```python
from build123d import *

# Parameters (mm, degrees)
F0_W     = 60
F0_H     = 60
F0_W_2   = 40.5
F0_H_2   = 31
F1_DEPTH = 3
F2_R     = 1.5
F3_DEPTH = 3.001
F4_W     = 40.5
F4_H     = 3
F5_DEPTH = 0.5
F6_R     = 1.6
F7_DEPTH = 3.001


with BuildPart() as f1:
    # F0 (on Top) → F1 (new body)
    with BuildSketch(Plane.XY):
        Rectangle(F0_W, F0_H)
        Rectangle(F0_W_2, F0_H_2, mode=Mode.SUBTRACT)
    extrude(amount=F1_DEPTH)

    # F2 (on face) → F3 (cut, through all)
    with BuildSketch(Plane.XY.offset(3)):
        with Locations((-25, -23)):
            Circle(F2_R)
        with Locations((-25, 23)):
            Circle(F2_R)
        with Locations((25, 23)):
            Circle(F2_R)
        with Locations((25, -23)):
            Circle(F2_R)
    extrude(amount=-F3_DEPTH, mode=Mode.SUBTRACT)

    # F4 (on face) → F5 (cut)
    with BuildSketch(Plane.XZ.offset(-15.5)):
        with Locations((0, 1.5)):
            Rectangle(F4_W, F4_H)
    extrude(amount=-F5_DEPTH, mode=Mode.SUBTRACT)

    # F6 (on face) → F7 (cut, through all)
    with BuildSketch(Plane.XY.offset(3)):
        with Locations((-25, 10)):
            Circle(F6_R)
        with Locations((-25, -17)):
            Circle(F6_R)
        with Locations((25, 10)):
            Circle(F6_R)
        with Locations((25, -17)):
            Circle(F6_R)
        with Locations((0, 23)):
            Circle(F6_R)
    extrude(amount=-F7_DEPTH, mode=Mode.SUBTRACT)


solid = f1.part
```
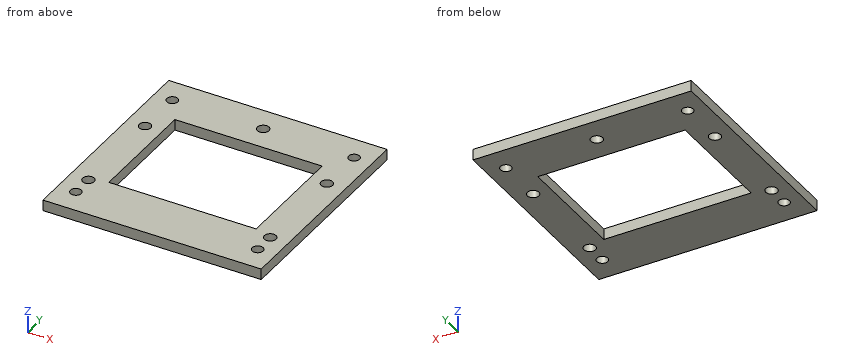
Part model, mm, in its own coordinate system. Coordinates: 2 decimals unless noted, no trailing zeros. Loops run counter-clockwise (first coordinate to the right, second up) from the corner with the lowest first, then second, coordinate; pieces in that order, holes last. Notation, with made-up numbers: (-11.5, -29) - (40.5, -29) arc R30 cw to (40.5, -1) - close; hole circle Ø6 at (-24, 24.25). An arc over 180 degrees is marked (long way). Write item = value, one per line. Start each with the question number.
Item 1: Cut at D-D, the plane x = 25. Give the cut face in (y, z).
Item 2: Cut at A-A, the plane y = 10. Give the cut face in (x, z), and give its area (3 significant figures).
Item 3: Wall check: L1, parallel to Y at x = 0, z = 2.2; L2, parallel to Y at x = 25, z = 1.75; L3, parallel to Y at x = -14, z = 2.45. Give the ranges that are in metal, low to high. Write a range as from..to.
Item 4: Flat gauge pin, fed straight in: pin 1 Ø6 at (x, y) = (-10, 21.5) entering from -Z. Where does the tip first touch, or does it go through?
Item 5: Cut at C-C, the plane y = -11.5. Give the cut face in (x, z).
Item 6: Cut at B-B, the plane x = 11.5. Give the cut face in (y, z), and give its area (3 significant figures).
The answers:
q1.outline = (-30, 0) - (-24.5, 0) - (-24.5, 3) - (-30, 3) - close; (-21.5, 0) - (-18.6, 0) - (-18.6, 3) - (-21.5, 3) - close; (-15.4, 0) - (8.4, 0) - (8.4, 3) - (-15.4, 3) - close; (11.6, 0) - (21.5, 0) - (21.5, 3) - (11.6, 3) - close; (24.5, 0) - (30, 0) - (30, 3) - (24.5, 3) - close
q2.outline = (-30, 0) - (-26.6, 0) - (-26.6, 3) - (-30, 3) - close; (-23.4, 0) - (-20.25, 0) - (-20.25, 3) - (-23.4, 3) - close; (20.25, 0) - (23.4, 0) - (23.4, 3) - (20.25, 3) - close; (26.6, 0) - (30, 0) - (30, 3) - (26.6, 3) - close
q2.area = 39.3 mm2
q3.L1 = -30..-15.5, 16..21.4, 24.6..30
q3.L2 = -30..-24.5, -21.5..-18.6, -15.4..8.4, 11.6..21.5, 24.5..30
q3.L3 = -30..-15.5, 16..30
q4.pin_1 = 0
q5.outline = (-30, 0) - (-20.25, 0) - (-20.25, 3) - (-30, 3) - close; (20.25, 0) - (30, 0) - (30, 3) - (20.25, 3) - close
q6.outline = (-30, 0) - (-15.5, 0) - (-15.5, 3) - (-30, 3) - close; (16, 0) - (30, 0) - (30, 3) - (16, 3) - close
q6.area = 85.5 mm2
